from build123d import *

# Parameters (mm, degrees)
F0_R     = 8.5
F0_R_2   = 6.985
F0_R_3   = 3.01878
F1_DEPTH = 10.16
F2_R     = 7.62
F3_DEPTH = 25.4


with BuildPart() as f1:
    # F0 (on Top) → F1 (new body)
    with BuildSketch(Plane.XY):
        with BuildLine():
            ThreePointArc((29.21, 104.385), (28.391776, 99.847507), (27.755027, 95.281012))
            ThreePointArc((27.755027, 95.281012), (28.843963, 99.77524), (29.21, 104.385))
        make_face()
        with BuildLine():
            ThreePointArc((89.287219, -21.055), (40.36409, 27.509427), (27.755027, 95.281012))
            ThreePointArc((27.755027, 95.281012), (28.391776, 99.847507), (29.21, 104.385))
            ThreePointArc((29.21, 104.385), (-7.560104, 132.599693), (-25.296602, 89.78))
            ThreePointArc((-25.296602, 89.78), (-42.893065, 23.129114), (-95.280447, -21.676448))
            ThreePointArc((-95.280447, -21.676448), (-99.553523, -23.408254), (-103.892219, -24.968398))
            ThreePointArc((-103.892219, -24.968398), (-109.941808, -70.919589), (-63.990617, -64.87))
            ThreePointArc((-63.990617, -64.87), (2.528975, -46.783541), (67.525421, -69.749564))
            ThreePointArc((67.525421, -69.749564), (71.161747, -72.584253), (74.682219, -75.561602))
            ThreePointArc((74.682219, -75.561602), (117.501913, -57.825104), (89.287219, -21.055))
        make_face()
        with Locations((-89.287219, -50.265)):
            Circle(F0_R, mode=Mode.SUBTRACT)
        Circle(F0_R_2, mode=Mode.SUBTRACT)
        with Locations((89.287219, -50.265)):
            Circle(F0_R_3, mode=Mode.SUBTRACT)
        with Locations((0, 104.385)):
            Circle(F0_R, mode=Mode.SUBTRACT)
        with BuildLine():
            ThreePointArc((67.525421, -69.749564), (70.873068, -72.939725), (74.682219, -75.561602))
            ThreePointArc((74.682219, -75.561602), (71.161747, -72.584253), (67.525421, -69.749564))
        make_face()
        with BuildLine():
            ThreePointArc((-103.892219, -24.968398), (-99.553523, -23.408254), (-95.280447, -21.676448))
            ThreePointArc((-95.280447, -21.676448), (-99.717031, -22.980515), (-103.892219, -24.968398))
        make_face()
    extrude(amount=F1_DEPTH)

    # F2
    f2_edges = [f1.edges().sort_by_distance(p)[0] for p in [
        (27.755027, 95.281012, 5.08),
        (-25.296602, 89.78, 5.08),
        (-63.990617, -64.87, 5.08),
        (-95.280447, -21.676448, 5.08),
        (67.525421, -69.749564, 5.08),
        (89.287219, -21.055, 5.08),
    ]]
    fillet(f2_edges, radius=F2_R)

    # F0 (on Top) → F3 (join)
    with BuildSketch(Plane.XY):
        with Locations((89.287219, -50.265)):
            Circle(F0_R_3)
    extrude(amount=F3_DEPTH)


solid = f1.part
Check sheet for the modelled part. Datum: model origin and axes. Units: mm. A direction names the side the tool comes from. Give positions to 0.01 mm unless a question says otherwise; leave off trailing zeros. Loops run counter-clockwise (first coordinate to the right, second up) from the corner with the lowest first, then second, coordinate; pieces in that order, holes last. Notation, with made-up numbers: M -20,-25 L 8,-25 A18 cw 8,-13 Z; hole C 82.5,13 d5. An arc over 180 degrees is marked long. Return JSON: item names as keys, results as strings. Group by question number.
1. Tool access check on faces 1 (the cylindrical face through (-42.672, 23.483, 5.009)), 2 (the cylindrical face through (71.078, -73.104, 5.009)), 3 (the cylindrical face through (86.89, -52.1, 17.67)), 4 (the cylindrical face through (28.884, 100.035, 5.009)), 5 (the cylindrical face through (-110.995, -69.81, 5.009)). Record the directions out of +Z, -Z, +X, -X, +Y, -Y that give a thin tool (end or side, any length) a straight path to the whole face; none if there is none.
2. Cross-section at D-D on y = 52.5. Record the boundary of the cut face in (x, z), plus the area to 3 significant figures.
3. Cross-section at B-B on y = 0. Record the boundary of the cut face in (x, z) (3 decimals), plus the area to 3 significant figures.
4. Cross-section at A-A on x = 0. Record the boundary of the cut face in (y, z) (3 decimals), plus the area to 3 significant figures.
5. Mould release check, pull along X, two halves, no side actions. Record for faces 6 (the cylindrical face through (-99.962, -23.075, 5.009)), 7 (the cylindrical face through (-97.78, -49.89, 5.01)), 8 (the flat face through (89, -50, 25.4)): released by +X, released by -X, zero draft, split by the parting line, or undercut.
6. Go/stop test with flat-tipped pins: pin 1 (3 mm diameter, centred on x = -3.5, y = 19.5, fed in from +Z); pin 2 (2 mm diameter, centred on y = -7, z = 3.5, fed in from +X); pin 3 (4 mm diameter, centred on y = -52, z = 16, fed in from -X). Record where each tip stops, or that it passes through.
7. Thickness scan on L1, parallel to Y at x = 0, z = 7.75 (3 decimals); L2, parallel to Z at x = -103, y = -37.5; L3, parallel to X at y = 70.5, z = 1. Record the ranges inside material, lowest first.
8. Cross-section at C-C on z = 4.5. State how many separate pieces and enclosed holes the cut face has, plus the area to 3 significant figures.
Return value:
{
 "1": {"face 1": "+Z, -Z, -X", "face 2": "+Z, -Z, -Y", "face 3": "+Z", "face 4": "+Z, -Z, +X", "face 5": "+Z, -Z"},
 "2": {"outline": "M -29.74,0 L 30.66,0 L 30.66,10.16 L -29.74,10.16 Z", "area": "614 mm^2"},
 "3": {"outline": "M -62.012,0 L -6.985,0 L -6.985,10.16 L -62.012,10.16 Z; M 6.985,0 L 60.621,0 L 60.621,10.16 L 6.985,10.16 Z", "area": "1,100 mm^2"},
 "4": {"outline": "M -46.717,0 L -6.985,0 L -6.985,10.16 L -46.717,10.16 Z; M 6.985,0 L 95.885,0 L 95.885,10.16 L 6.985,10.16 Z; M 112.885,0 L 133.595,0 L 133.595,10.16 L 112.885,10.16 Z", "area": "1,520 mm^2"},
 "5": {"face 6": "released by -X", "face 7": "undercut", "face 8": "zero draft"},
 "6": {"pin 1": "z = 10.16", "pin 2": "x = 69.45", "pin 3": "x = 86.27"},
 "7": {"L1": "-46.717 to -6.985, 6.985 to 95.885, 112.885 to 133.595", "L2": "0 to 10.16", "L3": "-26.05 to 27.48"},
 "8": {"separate pieces": "1", "enclosed holes": "3", "area": "20,700 mm^2"}
}
